Check sheet for the modelled part. Datum: model origin and axes. Units: mm. Face numbers are marked on the shaded views. A direction names the side the tool comes from. Coordinates: 2 decimals unless noted, no trailing zeros. Write each loop counter-clockwise with the first axis right and the second up, starting at its lowest first coordinate (ties: lowest second). Pieces come first, ordered by that corner, then holes. Notation, with made-up numbers: M 74,12.5 L 121,12.5 A13 ccw 121,34.5 Z; hole C -23,41.25 d10. An arc over 180 degrees is marked long. Answer as CSV lines item,"result".
from build123d import *

# Parameters (mm, degrees)
CHAMFER1_SIZE      = 1.5
CUT_EXTRUDE1_DEPTH = 8


with BuildPart() as part:
    # Sketch1 → Revolve1 (revolve)
    with BuildSketch(Plane.XY, mode=Mode.PRIVATE) as revolve1_sk:
        Polygon((0, 0), (4.5, 0), (4.5, 11.5), (6, 11.5), (6, 55), (10.5, 55), (10.5, 70), (0, 70), align=None)
    revolve(revolve1_sk.sketch.rotate(Axis((0, 70, 0), (0, -1, 0)), 180), axis=Axis((0, 70, 0), (0, -1, 0)))

    # Chamfer1
    chamfer1_edges = [part.edges().sort_by_distance(p)[0] for p in [
        (10.5, 70, 0),
        (10.5, 55, 0),
        (6, 11.5, 0),
    ]]
    chamfer(chamfer1_edges, length=CHAMFER1_SIZE - 0.0001)  # a hair under: the kernel refuses the full size

    # Sketch2 → Cut-Extrude1 (cut)
    with BuildSketch(Plane(origin=(0, 70, 0), x_dir=(1, 0, 0), z_dir=(0, 1, 0))):
        Polygon((0, 4.618802154), (-4, 2.309401077), (-4, -2.309401077), (0, -4.618802154), (4, -2.309401077), (4, 2.309401077), align=None)
    extrude(amount=-CUT_EXTRUDE1_DEPTH, mode=Mode.SUBTRACT)


solid = part.part
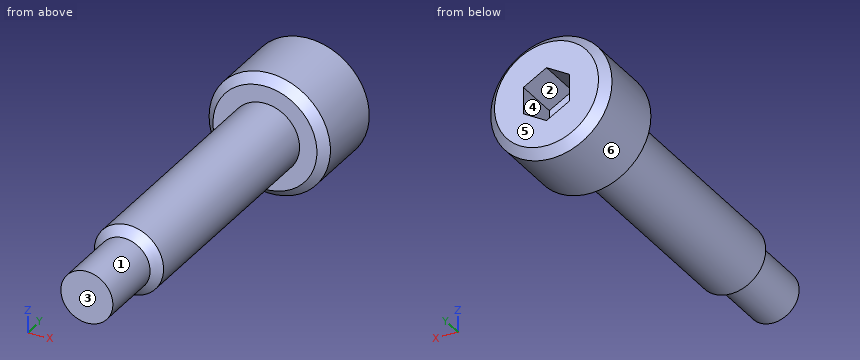
1) Section check C-C, the plane y = 32.5. Record the boundary of the cut face in (x, z), plus the area to 3 significant figures.
Answer key:
outline,"C 0,0 d12"
area,"113 mm2"
2) Tool access check on the marked faces 1, 2 and 3. Record the directions out of +Z, -Z, +X, -X, +Y, -Y that give a thin tool (end or side, any length) a straight path to the whole face; none if there is none.
Answer key:
face 1,"-Y"
face 2,"+Y"
face 3,"+Z, -Z, +X, -X, -Y"
3) Depth check by flat-ended pin: P1, Ø8, axis at x = 3.5, y = 58.5, coming from the -Z side; P2, Ø5, axis at x = -4, y = 31, coming from the +Z side; P3, Ø8, axis at y = 32, z = -7, coming from the +X side; P4, Ø4, axis at x = 0, z = -0.5, coming from the +Y side. Enter the tip coordinate at first touch or a pass-through.
Answer key:
P1,"stops at z = -10.5"
P2,"stops at z = 5.81"
P3,"stops at x = 5.2"
P4,"stops at y = 62"
4) Section check A-A, the plane y = 63.5. Record the boundary of the cut face in (x, z).
Answer key:
outline,"C 0,0 d21; hole M -4,-2.31 L 0,-4.62 L 4,-2.31 L 4,2.31 L 0,4.62 L -4,2.31 Z"
5) Mould release check, pull along X, two halves, no side actions. Record for the marked faces 4, 5 and 6: pulls with the +X half, pulls with the -X half, needs draft (parallel to the pull), parting line crosses it, or undercut.
Answer key:
face 4,"undercut"
face 5,"needs draft"
face 6,"parting line crosses it"
6) Thickness scan on line 1 along Y through (x, z) = (-3.75, -5); line 2 along X through (y, z) = (65, -0.5); line 3 along Z through (x, y) = (0, 5). Record the ranges inside material, lowest first.
Answer key:
line 1,"y = 55 to 70"
line 2,"x = -10.49 to -4, 4 to 10.49"
line 3,"z = -4.5 to 4.5"
